from build123d import *

# Parameters (mm, degrees)
F0_W     = 58
F0_H     = 67
F1_DEPTH = 10
F2_R     = 3
F2_R_2   = 6
F3_DEPTH = 25
F4_SIZE  = 3


with BuildPart() as f1:
    # F0 (on Top) → F1 (new body)
    with BuildSketch(Plane.XY):
        Polygon((-40, -95), (40, -95), (40, -28), (40, 95), (-40, 95), align=None)
        with Locations((69, -61.5)):
            Rectangle(F0_W, F0_H)
    extrude(amount=F1_DEPTH)

    # F2 (on face) → F3 (cut)
    with BuildSketch(Plane.XY.offset(10)):
        with Locations((48, -78)):
            Circle(F2_R)
        with Locations((48, -42)):
            Circle(F2_R)
        with Locations((69, -78)):
            Circle(F2_R)
        with Locations((69, -42)):
            Circle(F2_R)
        with Locations((-15, 63)):
            Circle(F2_R_2)
        with Locations((15, 25)):
            Circle(F2_R_2)
    extrude(amount=-F3_DEPTH, mode=Mode.SUBTRACT)

    # F4
    f4_edges = [f1.edges().sort_by_distance(p)[0] for p in [
        (66, -78, 0),
        (45, -78, 0),
        (45, -42, 0),
        (66, -42, 0),
    ]]
    chamfer(f4_edges, length=F4_SIZE)


solid = f1.part
Work out the finished part from the listing and answer in its coordinate system (mm). A direction names the side the tool comes from. Give positions to 0.01 mm unless a question says otherwise; leave off trailing zeros. Loops run counter-clockwise (first coordinate to the right, second up) from the corner with the lowest first, then second, coordinate; pieces in that order, holes last. Notation, with made-up numbers: (51.25, 12) - (59.25, 12) arc R22 ccw to (59.25, 32) - close; hole circle Ø4 at (49, -6). An arc over 180 degrees is marked (long way). Answer in a Markdown table with one row per item. Add a question column.
Q1. The part is cut by section B-B (z = 7). Determine the outline of the cut face in (x, y), and give its area (3 significant figures).
Q2. Each of these flat-tipped pins is pushed along its axis until it touches: P1, Ø3, axis at y = 26.5, z = 3, coming from the +X side; P2, Ø3.5, axis at x = 48, y = -42, coming from the +Z side; P3, Ø9.5, axis at x = 48, y = -78, coming from the -Z side; P4, Ø2, axis at x = 49, z = 1, coming from the +Y side. Where does it stop, or does it pass through?
Q3. Determine the mould class of faces 3 (the flat face through (28, -95, 5)), 4 (the conical face through (70.452, -44.791, 2.854)), 5 (the flat face through (40, 33, 5)) for opening direction X: released by +X, released by -X, zero draft, split by the parting line, or undercut.
Q4. The part is cut by section C-C (y = -42). Determine the outline of the cut face in (x, z).
Q5. The part is cut by section D-D (x = -15). Determine the outline of the cut face in (y, z).
Q6. A tool of negligible diameter and unlimited length cuts with its end or side. For faces 1 (the flat face through (13, -20, 0)), 2 (the flat face through (69, -28, 5)), from which of +Z, -Z, +X, -X, +Y, -Y can it reach the whole face along a straight path? Write none if from no direction.
Q7. Consider line 1 along Y through (x, z) = (69, 4.75); line 2 along Y through (x, z) = (15, 2); line 3 along X through (y, z) = (52, 2.5). Determine where each line is inside the solid, lowest interval first.
Q8. The part is cut by section A-A (x = 69). Determine the outline of the cut face in (y, z), and give its area (3 significant figures).
Solution:
| question | item | result |
|---|---|---|
| 1 | outline | (-40, -95) - (98, -95) - (98, -28) - (40, -28) - (40, 95) - (-40, 95) - close; hole circle Ø12 at (-15, 63); hole circle Ø12 at (15, 25); hole circle Ø6 at (48, -78); hole circle Ø6 at (48, -42); hole circle Ø6 at (69, -78); hole circle Ø6 at (69, -42) |
| 1 | area | 18,700 mm² |
| 2 | P1 | stops at x = 40 |
| 2 | P2 | passes through |
| 2 | P3 | stops at z = 1.25 |
| 2 | P4 | stops at y = -28 |
| 3 | face 3 | zero draft |
| 3 | face 4 | undercut |
| 3 | face 5 | released by +X |
| 4 | outline | (-40, 0) - (42, 0) - (45, 3) - (45, 10) - (-40, 10) - close; (51, 3) - (54, 0) - (63, 0) - (66, 3) - (66, 10) - (51, 10) - close; (72, 3) - (75, 0) - (98, 0) - (98, 10) - (72, 10) - close |
| 5 | outline | (-95, 0) - (57, 0) - (57, 10) - (-95, 10) - close; (69, 0) - (95, 0) - (95, 10) - (69, 10) - close |
| 6 | face 1 | -Z, +X, -X, +Y, -Y |
| 6 | face 2 | +Z, -Z, +X, +Y |
| 7 | line 1 | y = -95 to -81, -75 to -45, -39 to -28 |
| 7 | line 2 | y = -95 to 19, 31 to 95 |
| 7 | line 3 | x = -40 to 40 |
| 8 | outline | (-95, 0) - (-84, 0) - (-81, 3) - (-81, 10) - (-95, 10) - close; (-75, 3) - (-72, 0) - (-48, 0) - (-45, 3) - (-45, 10) - (-75, 10) - close; (-39, 3) - (-36, 0) - (-28, 0) - (-28, 10) - (-39, 10) - close |
| 8 | area | 532 mm² |
